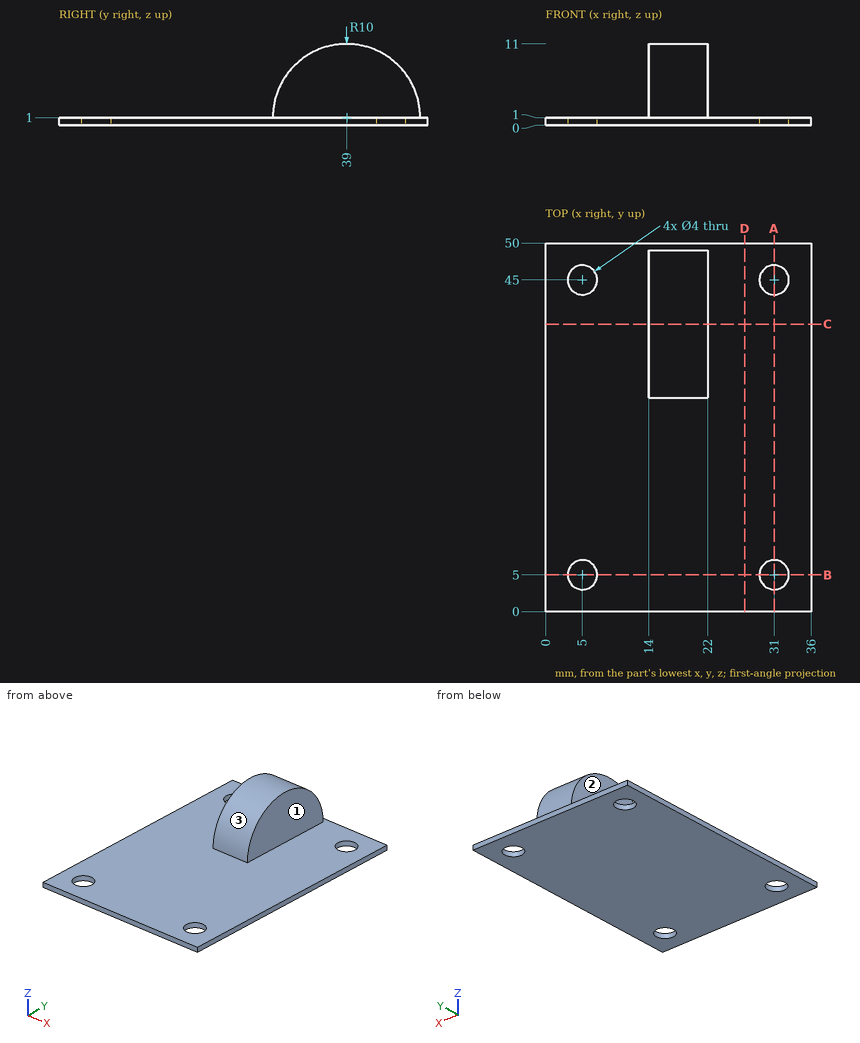
Input: dimensioned drawing with shaded views. Units: mm. Origin: part minimum x, y, z. A direction names the side the tool comes from. Give positions to 0.01 mm unless a question says otherwise; leave off trailing zeros. Write each loop counter-clockwise with the first axis right and the second up, starting at its lowest first coordinate (ties: lowest second). Pieces come first, ordered by that corner, then holes.
1. Material intervals for line 1 along Y through (x, z) = (5, 0.6); line 2 along Z through (x, y) = (7, 46.5); line 3 along X through (y, z) = (36.5, 3), sorted ascending.
2. Section query C-C (y = 39). Return the cut outline in (x, z).
3. Section query D-D (x = 27). Return the cut outline in (y, z).
4. Access query for the marked faces 1, 2 and 3. Directions: +Z, -Z, +X, -X, +Y, -Y. A direction counts if a zero-diameter tool reaches every point of the face in a straight line with its end or side. Return the directions, or none.
5. First-contact query: pin 1 (5 mm diameter, centred on x = 31, y = 5, fed in from +Z); pin 2 (1.5 mm diameter, centred on y = 8, z = 3, fed in from -X); pin 3 (3 mm diameter, centred on y = 40, z = 6.5, fed in from -X). Flat tips, straight axial feed; report the tip coordinate or a pass-through.
6. Section query A-A (x = 31). Return the cut outline in (y, z), then the cut area to 3 significant figures.
7. Section query B-B (y = 5). Return the cut outline in (x, z).
Output values:
1. line 1: y = 0 to 3, 7 to 43, 47 to 50
1. line 2: z = 0 to 1
1. line 3: x = 14 to 22
2. outline: (0, 0) - (36, 0) - (36, 1) - (22, 1) - (22, 11) - (14, 11) - (14, 1) - (0, 1) - close
3. outline: (0, 0) - (50, 0) - (50, 1) - (0, 1) - close
4. face 1: +Z, +X, +Y, -Y
4. face 2: +Z, -X, +Y, -Y
4. face 3: +Z, +X, -X
5. pin 1: stops at z = 1
5. pin 2: passes through
5. pin 3: stops at x = 14
6. outline: (0, 0) - (3, 0) - (3, 1) - (0, 1) - close; (7, 0) - (43, 0) - (43, 1) - (7, 1) - close; (47, 0) - (50, 0) - (50, 1) - (47, 1) - close
6. area: 42.0 mm2
7. outline: (0, 0) - (3, 0) - (3, 1) - (0, 1) - close; (7, 0) - (29, 0) - (29, 1) - (7, 1) - close; (33, 0) - (36, 0) - (36, 1) - (33, 1) - close
